```python
from build123d import *

# Parameters (mm, degrees)
F1_DEPTH = 63.5
F2_DEPTH = 25.4
F3_DEPTH = 12.7
F5_R     = 5.08


with BuildPart() as f1:
    # F0 (on Front) → F1 (new body, symmetric)
    with BuildSketch(Plane.XZ):
        Polygon((41.275, -9.525), (41.275, 9.525), (20.8620596677, 9.525), (-41.275, 9.525), (-41.275, -9.525), align=None)
    extrude(amount=F1_DEPTH, both=True)

    # F0 (on Front) → F2 (join, symmetric)
    with BuildSketch(Plane.XZ):
        with BuildLine():
            Line((20.8620596677, 9.525), (41.275, 9.525))
            Line((41.275, 9.525), (41.275, 27.0139881611))
            ThreePointArc((41.275, 27.0139881611), (46.1610443741, 38.4707974574), (57.8115013232, 42.8752))
            Line((57.8115013232, 42.8752), (60.325, 42.8752))
            Line((60.325, 42.8752), (60.325, 63.2881403323))
            Line((60.325, 63.2881403323), (56.1497511215, 63.2881403323))
            add(Edge.make_bspline(
                [(55.8418284891, 63.2783411935), (55.9444554247, 63.281668613), (56.0470964076, 63.2849348987), (56.1497511215, 63.2881403323)],
                knots=[111.0026419847, 111.0026419847, 111.0026419847, 111.0026419847, 111.2746933919, 111.2746933919, 111.2746933919, 111.2746933919], degree=3))
            ThreePointArc((55.8418284891, 63.2783411935), (31.03213769, 52.206683172), (20.8620596677, 27.0139881611))
            Line((20.8620596677, 27.0139881611), (20.8620596677, 9.525))
        make_face()
        Polygon((60.325, 63.2881403323), (60.325, 42.8752), (85.725, 42.8752), (85.725, 52.3875), (85.725, 63.2881403323), align=None)
    extrude(amount=F2_DEPTH, both=True)

    # F0 (on Front) → F3 (join, symmetric)
    with BuildSketch(Plane.XZ):
        with BuildLine():
            Line((-41.275, 9.525), (20.8620596677, 9.525))
            Line((20.8620596677, 9.525), (20.8620596677, 27.0139881611))
            ThreePointArc((20.8620596677, 27.0139881611), (31.03213769, 52.206683172), (55.8418284891, 63.2783411935))
            add(Edge.make_bspline(
                [(-41.275, 9.525), (-25.5674248784, 50.3853946243), (13.9679006475, 61.920684693), (55.8418284891, 63.2783411935)],
                knots=[0, 0, 0, 0, 111.0026419847, 111.0026419847, 111.0026419847, 111.0026419847], degree=3))
        make_face()
    extrude(amount=F3_DEPTH, both=True)

    # F0 (on Front) → F4 (revolve)
    with BuildSketch(Plane.XZ):
        Polygon((85.725, 52.3875), (85.725, 42.8752), (85.725, 38.1), (111.125, 38.1), (111.125, 66.675), (85.725, 66.675), (85.725, 63.2881403323), align=None)
    revolve(axis=Axis((85.725, 0, 54.7751), (0, 0, 1)))

    # F5
    f5_edges = [f1.edges().sort_by_distance(p)[0] for p in [
        (41.275, -63.5, 0),
        (-41.275, -63.5, 0),
        (-41.275, 63.5, 0),
        (41.275, 63.5, 0),
    ]]
    fillet(f5_edges, radius=F5_R)


solid = f1.part
```
Build history of the part. All positions in model axes, mm. A direction names the side the tool comes from. Give positions to 0.01 mm unless a question says otherwise; leave off trailing zeros. Loops run counter-clockwise (first coordinate to the right, second up) from the corner with the lowest first, then second, coordinate; pieces in that order, holes last.
Item 1: Drill centre lines: line 1 (Z direction, x = 26, y = 37.5) (3 decimals); line 2 (Y direction, x = -16, z = 40); line 3 (Z direction, x = 73, y = -11) (3 decimals). Where is each one in solid material? Low to high.
Answers follow:
line 1: z = -9.525 to 9.525
line 2: y = -12.7 to 12.7
line 3: z = 38.1 to 66.675
Item 2: Slice it at C-C, the plane y = 47.5. List the corners of the cut face in (x, z) (3 decimals).
Answers follow:
outline: (-41.275, -9.525) - (41.275, -9.525) - (41.275, 9.525) - (-41.275, 9.525) - close
Item 3: Flat gauge pins, fed straight in: pin 1 (11 mm diameter, centred on y = 21.5, z = 11.5, fed in from +X) (3 decimals); pin 2 (4 mm diameter, centred on y = -17.5, z = 14, fed in from -X); pin 3 (15 mm diameter, centred on x = 12.5, y = 49.5, fed in from +Z) (3 decimals). Where does each tip first touch, or does it go through?
Answers follow:
pin 1: stops at x = 41.275
pin 2: stops at x = 20.86
pin 3: stops at z = 9.525
Item 4: Which spindle directions (+Z, -Z, +X, -X, +Y, -Y) get a long thin tool onto all of the face, cutting with end or side? Do faces 1 (the face through (20.862, -19, 18)), 2 (the face through (60, 0, 63.288)), 3 (the face through (46, 25.4, 43)), 4 (the face through (31.304, 18.961, 52.486)). Say none if no direction does.
Answers follow:
face 1: +Z, -X, -Y
face 2: +Z, -X
face 3: +Z, +X, -X, +Y
face 4: +Z, -X, +Y
Item 5: Slice it at A-A, the plane z = 4. List the corners of the cut face in (x, y) (3 decimals), and give its area (3 significant figures).
Answers follow:
outline: (-41.275, -58.42) arc R5.08 ccw to (-36.195, -63.5) - (36.195, -63.5) arc R5.08 ccw to (41.275, -58.42) - (41.275, 58.42) arc R5.08 ccw to (36.195, 63.5) - (-36.195, 63.5) arc R5.08 ccw to (-41.275, 58.42) - close
area: 10,500 mm2
Item 6: Slice it at B-B, the plane x = 84. List the corners of the cut face in (y, z) (3 decimals).
Answers follow:
outline: (-25.4, 42.875) - (-25.341, 42.875) - (-25.341, 38.1) - (25.341, 38.1) - (25.341, 42.875) - (25.4, 42.875) - (25.4, 63.288) - (25.341, 63.288) - (25.341, 66.675) - (-25.341, 66.675) - (-25.341, 63.288) - (-25.4, 63.288) - close
